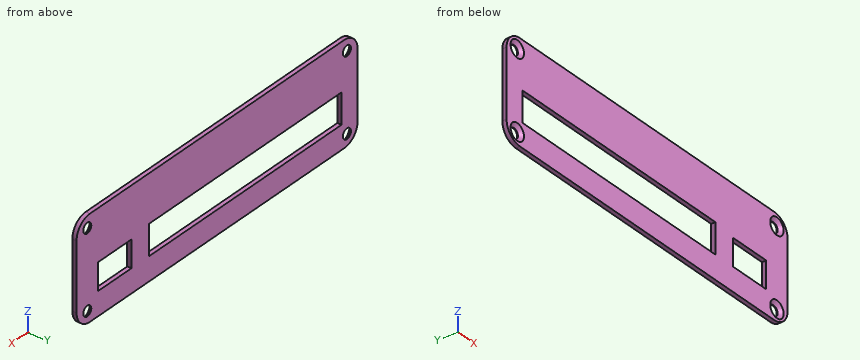
```python
from build123d import *

# Parameters (mm, degrees)
F0_W     = 105
F0_H     = 30
F0_R     = 1.5
F0_W_2   = 72
F0_H_2   = 9
F0_W_3   = 12.5
F0_H_3   = 8
F1_DEPTH = 1.25
F2_R     = 5
F3_SIZE  = 1


with BuildPart() as f1:
    # F0 (on Front) → F1 (new body)
    with BuildSketch(Plane.XZ):
        with Locations((16.557691, -4.707695)):
            Rectangle(F0_W, F0_H)
        with Locations((-31.942309, -16.207695)):
            Circle(F0_R, mode=Mode.SUBTRACT)
        with Locations((6.057691, -8.207695)):
            Rectangle(F0_W_2, F0_H_2, mode=Mode.SUBTRACT)
        with Locations((65.057691, -16.207695)):
            Circle(F0_R, mode=Mode.SUBTRACT)
        with Locations((54.807691, -8.707695)):
            Rectangle(F0_W_3, F0_H_3, mode=Mode.SUBTRACT)
        with Locations((-31.942309, 6.792305)):
            Circle(F0_R, mode=Mode.SUBTRACT)
        with Locations((65.057691, 6.792305)):
            Circle(F0_R, mode=Mode.SUBTRACT)
    extrude(amount=F1_DEPTH)

    # F2
    f2_edges = [f1.edges().sort_by_distance(p)[0] for p in [
        (69.057691, -0.625, 10.292305),
        (69.057691, -0.625, -19.707695),
        (-35.942309, -0.625, -19.707695),
        (-35.942309, -0.625, 10.292305),
    ]]
    fillet(f2_edges, radius=F2_R)

    # F3
    f3_edges = [f1.edges().sort_by_distance(p)[0] for p in [
        (-33.442309, -1.25, 6.792305),
        (-33.442309, -1.25, -16.207695),
        (63.557691, -1.25, -16.207695),
        (63.557691, -1.25, 6.792305),
    ]]
    chamfer(f3_edges, length=F3_SIZE)


solid = f1.part
```
Design review of the part built by this model. Coordinates are the model's own, in mm. Round coordinates to 2 decimals unless told otherwise and drop trailing zeros. Order: outer loops, then holes, each group sorted by start corner. A loop starts at its lowest first (then second) coordinate and runs counter-clockwise, first axis right, second up. Notation, with made-up numbers: M 20,8.25 L 40,8.25 A19 cw 40,27.25 Z; hole C 70.25,57.25 d1. An arc over 180 degrees is marked long. Put each result on its own line as item: value.
Q1. To check wall thickness, follow line 1 (X direction, y = -0.15, z = -11); line 2 (Z direction, x = 35, y = -0.95); line 3 (X direction, y = -0.2, z = 6.25). State the ranges of each line that lie inside material, in increasing order.
Reported:
line 1: -35.94 to -29.94, 42.06 to 48.56, 61.06 to 69.06
line 2: -19.71 to -12.71, -3.71 to 10.29
line 3: -35.85 to -33.34, -30.54 to 63.66, 66.46 to 68.97
Q2. Consider section C-C (y = -0.8). State the section outline as (x, z) points, and give its area (3 significant figures).
Reported:
outline: M -35.94,-14.71 A5 ccw -30.94,-19.71 L 64.06,-19.71 A5 ccw 69.06,-14.71 L 69.06,5.29 A5 ccw 64.06,10.29 L -30.94,10.29 A5 ccw -35.94,5.29 Z; hole C -31.94,-16.21 d4.1; hole C -31.94,6.79 d4.1; hole M -29.94,-12.71 L 42.06,-12.71 L 42.06,-3.71 L -29.94,-3.71 Z; hole M 48.56,-12.71 L 61.06,-12.71 L 61.06,-4.71 L 48.56,-4.71 Z; hole C 65.06,-16.21 d4.1; hole C 65.06,6.79 d4.1
area: 2,330 mm²
Q3. Consider section A-A (z = -11). State the section outline as (x, y) points, and give its area (3 significant figures).
Reported:
outline: M -35.94,-1.25 L -29.94,-1.25 L -29.94,0 L -35.94,0 Z; M 42.06,-1.25 L 48.56,-1.25 L 48.56,0 L 42.06,0 Z; M 61.06,-1.25 L 69.06,-1.25 L 69.06,0 L 61.06,0 Z
area: 25.6 mm²
Q4. Consider section B-B (x = -8.5). State the section outline as (y, z) points, and give its area (4 significant figures).
Reported:
outline: M -1.25,-19.71 L 0,-19.71 L 0,-12.71 L -1.25,-12.71 Z; M -1.25,-3.71 L 0,-3.71 L 0,10.29 L -1.25,10.29 Z
area: 26.25 mm²
Q5. Insertion check: pin 1 Ø4 at (x, z) = (46.5, -2) entering from +Y; pin 2 Ø4 at (x, z) = (65.06, 6.79) entering from -Y. Each pin has a flat end and moves straight along its axis. Give the tip position at first contact, or say it passes through.
Reported:
pin 1: y = 0
pin 2: y = -0.75
